from build123d import *

# Parameters (mm, degrees)
SKETCH_W        = 12.7
SKETCH_H        = 88.9
PAD_DEPTH       = 587.3
SKETCH001_W     = 6.35
SKETCH001_H     = 12.7
POCKET_DEPTH    = 587.301
SKETCH002_W     = 6.35
SKETCH002_H     = 6.35
POCKET001_DEPTH = 88.901


with BuildPart() as part:
    # Sketch → Pad (new body)
    with BuildSketch(Plane.YZ):
        with Locations((6.35, 44.45)):
            Rectangle(SKETCH_W, SKETCH_H)
    extrude(amount=PAD_DEPTH)

    # Sketch001 (on Face6 of Pad) → Pocket (cut, through all)
    with BuildSketch(Plane.YZ.offset(587.3)):
        with Locations((9.525, 12.7)):
            Rectangle(SKETCH001_W, SKETCH001_H)
    extrude(amount=-POCKET_DEPTH, mode=Mode.SUBTRACT)

    # Sketch002 (on Face6 of Pocket) → Pocket001 (cut, through all)
    with BuildSketch(Plane(origin=(0, 0, 88.9), x_dir=(0, -1, 0), z_dir=(0, 0, 1))):
        with Locations((-9.525, 584.125)):
            Rectangle(SKETCH002_W, SKETCH002_H)
        with Locations((-9.525, 3.175)):
            Rectangle(SKETCH002_W, SKETCH002_H)
    extrude(amount=-POCKET001_DEPTH, mode=Mode.SUBTRACT)


solid = part.part
CAD build for the part. Positions are in the model's coordinates, mm. Round coordinates to 2 decimals unless told otherwise and drop trailing zeros. Loops run counter-clockwise (first coordinate to the right, second up) from the corner with the lowest first, then second, coordinate; pieces in that order, holes last. Notation, with made-up numbers: M -27.75,-38 L 24.25,-38 A27 cw 24.25,-16 Z; hole C 33.25,25.25 d11. An arc over 180 degrees is marked long. One line per question, with ' | ' between items. Start each with the question number.
Item 1: Cut at C-C, the plane z = 13.5. Write the cut outline in (x, y).
Item 2: Two-plate mould, pull along Z, no slides. Class faces 1 (the flat face through (290, 12.7, 53)), 2 (the flat face through (290, 6, 88.9)), 3 (the flat face through (292, 6.35, 15)), 4 (the flat face through (290, 6, 0)): pulls with the +Z half, pulls with the -Z half, needs draft (parallel to the pull), parting line crosses it, or undercut.
Item 3: Pin check, flat tip, straight feed: pin 1 Ø4 at (y, z) = (9, 32.5) entering from -X. Stop position of the tip, or through.
Item 4: Cut at A-A, the plane y = 9.5. Write the cut outline in (x, z), plus the area to 3 significant figures.
Item 5: Cut at B-B, the plane x = 99.5. Write the cut outline in (y, z), plus the area to 3 significant figures.
Item 6: Wall check: line 1 (Z direction, x = 57, y = 10); line 2 (X direction, y = 8.75, z = 74); line 3 (Y direction, x = 530, z = 11.5). Give the ranges that are in metal, low to high.
Responses:
1) outline: M 0,0 L 587.3,0 L 587.3,6.35 L 0,6.35 Z
2) face 1: needs draft | face 2: pulls with the +Z half | face 3: undercut | face 4: pulls with the -Z half
3) pin 1: stops at x = 6.35
4) outline: M 6.35,0 L 580.95,0 L 580.95,6.35 L 6.35,6.35 Z; M 6.35,19.05 L 580.95,19.05 L 580.95,88.9 L 6.35,88.9 Z | area: 43,800 mm²
5) outline: M 0,0 L 12.7,0 L 12.7,6.35 L 6.35,6.35 L 6.35,19.05 L 12.7,19.05 L 12.7,88.9 L 0,88.9 Z | area: 1,050 mm²
6) line 1: z = 0 to 6.35, 19.05 to 88.9 | line 2: x = 6.35 to 580.95 | line 3: y = 0 to 6.35
